Input: part model. Units: mm. Frame: model coordinates. A direction names the side the tool comes from. Give positions to 0.01 mm unless a question says otherwise; leave off trailing zeros. Write each loop counter-clockwise with the first axis right and the second up, starting at its lowest first coordinate (ties: lowest second). Pieces come first, ordered by that corner, then holes. Notation, with made-up numbers: (-20, 39.25) - (35, 39.25) arc R18 cw to (35, 50.25) - close; hole circle Ø10 at (57, 30.25). An arc over 180 degrees is marked (long way). Answer as a JSON object with one key per item and string values. Group by question number.
from build123d import *

# Parameters (mm, degrees)
BOSS_EXTRUDE1_DEPTH = 2.5
SKETCH5_W           = 2.85
SKETCH5_H           = 2.5
CUT_EXTRUDE3_DEPTH  = 10
SKETCH6_W           = 2.85
SKETCH6_H           = 2.5
CUT_EXTRUDE4_DEPTH  = 10
SKETCH7_W           = 2.85
SKETCH7_H           = 2.5
CUT_EXTRUDE5_DEPTH  = 10


with BuildPart() as part:
    # Sketch1 → Boss-Extrude1 (new body)
    with BuildSketch(Plane(origin=(0, 0, 0), x_dir=(1, 0, 0), z_dir=(0, 1, 0))):
        Polygon((11.547005384, 0), (5.773502692, 10), (-5.773502692, 10), (-11.547005384, 0), (-5.773502692, -10), (5.773502692, -10), align=None)
    extrude(amount=BOSS_EXTRUDE1_DEPTH)

    # Sketch5 → Cut-Extrude3 (cut)
    with BuildSketch(Plane.XY.offset(10)):
        with Locations((-4.348502692, 1.25)):
            Rectangle(SKETCH5_W, SKETCH5_H)
    extrude(amount=-CUT_EXTRUDE3_DEPTH, mode=Mode.SUBTRACT)

    # Sketch6 → Cut-Extrude4 (cut)
    with BuildSketch(Plane.XY.offset(10)):
        with Locations((4.348502692, 1.25)):
            Rectangle(SKETCH6_W, SKETCH6_H)
    extrude(amount=-CUT_EXTRUDE4_DEPTH, mode=Mode.SUBTRACT)

    # Sketch7 → Cut-Extrude5 (cut)
    with BuildSketch(Plane(origin=(0, 0, -10), x_dir=(-1, 0, 0), z_dir=(0, 0, -1))):
        with Locations((-0.011497308, 1.25)):
            Rectangle(SKETCH7_W, SKETCH7_H)
    extrude(amount=-CUT_EXTRUDE5_DEPTH, mode=Mode.SUBTRACT)


solid = part.part
1) Mould query, pull axis X, two halves, no side actions, for faces 1 (the face through (8.62, 1.23, 5.07)), 2 (the face through (2, 2.5, 0)), 3 (the face through (-8.7, 1.23, 4.93)), 4 (the face through (0, 1, 0)). Classes: +X half, -X half, draft (parallel to the pull), parting line (faces both ways), or undercut.
2) Cut plane B-B on z = -3. Return the cut outline in (x, y).
3) Pin query (flat end, axial travel): P1, Ø0.8, axis at y = 1, z = -5, coming from the -X side; P2, Ø0.8, axis at y = 1.5, z = 5.5, coming from the +X side; P3, Ø1.2, axis at x = 4, y = 0.5, coming from the +Z side. Return the tip coordinate at first contact, or that it passes through.
4) Cut plane C-C on z = 5.25. Return the cut outline in (x, y), and give its area (3 significant figures).
5) Line query: line 1 along X through (y, z) = (1.2, 3.75); line 2 along X through (y, z) = (0.6, 8); line 3 along Z through (x, y) = (-0.5, 1.85). Output: solid intervals per line, ascending. Write a range as from..to.
6) Cut plane A-A on y = 2.2. Return the cut outline in (x, z).
7) Reachability of faces 5 (the face through (1.436, 1, -5)), 6 (the face through (-4, 1, -10)), 7 (the face through (-2.924, 1, 5)) from +Z, -Z, +X, -X, +Y, -Y: full face, straight path, thin tool, end or side. Return the list, or none.
8) Cut plane D-D on x = -3.5. Return the cut outline in (y, z).
Filled in:
{
 "1": {"face 1": "+X half", "face 2": "draft", "face 3": "-X half", "face 4": "undercut"},
 "2": {"outline": "(-9.81, 0) - (-1.41, 0) - (-1.41, 2.5) - (-9.81, 2.5) - close; (1.44, 0) - (9.81, 0) - (9.81, 2.5) - (1.44, 2.5) - close"},
 "3": {"P1": "stops at x = -8.89", "P2": "stops at x = 8.6", "P3": "stops at z = 0"},
 "4": {"outline": "(-8.52, 0) - (-5.77, 0) - (-5.77, 2.5) - (-8.52, 2.5) - close; (-2.92, 0) - (2.92, 0) - (2.92, 2.5) - (-2.92, 2.5) - close; (5.77, 0) - (8.52, 0) - (8.52, 2.5) - (5.77, 2.5) - close", "area": "28.3 mm²"},
 "5": {"line 1": "x = -9.38..-5.77, -2.92..2.92, 5.77..9.38", "line 2": "x = -6.93..-5.77, -2.92..2.92, 5.77..6.93", "line 3": "z = 0..10"},
 "6": {"outline": "(-11.55, 0) - (-5.77, -10) - (-1.41, -10) - (-1.41, 0) - (1.44, 0) - (1.44, -10) - (5.77, -10) - (11.55, 0) - (5.77, 10) - (5.77, 0) - (2.92, 0) - (2.92, 10) - (-2.92, 10) - (-2.92, 0) - (-5.77, 0) - (-5.77, 10) - close"},
 "7": {"face 5": "-Z, +Y, -Y", "face 6": "-Z, +X, -X, +Y, -Y", "face 7": "+Z, +Y, -Y"},
 "8": {"outline": "(0, -10) - (2.5, -10) - (2.5, 0) - (0, 0) - close"}
}
